The figure shows three views and two pictorial views of one solid part (mm, origin at its lowest corner). Answer the questions. A direction names the side the tool comes from. Coordinates: 2 decimals unless noted, no trailing zeros. Loops run counter-clockwise (first coordinate to the right, second up) from the corner with the lowest first, then second, coordinate; pieces in that order, holes last. Notation, with made-up numbers: M -20.75,65.5 L 6.25,65.5 A28 cw 6.25,89.5 Z; hole C -4,6.25 d9. An arc over 180 degrees is marked long. Return JSON: item names as keys, results as strings. Group by question number.
1. The mould has two halves that part along X. Classify the marked faces 1, 2 and 3: pulls with the +X half, pulls with the -X half, needs draft (parallel to the pull), parting line crosses it, or undercut.
2. Which of the six approach directions +Z, -Z, +X, -X, +Y, -Y give full straight-line access (tool end or side, diameter ignored) to the marked faces 4, 5, 6, 7 and 8?
3. Straight lines are drawn through the part: L1, parallel to X at y = 5.75, z = 1 (1 decimal); L2, parallel to Z at x = 3, y = 4.75; L3, parallel to Y at x = 9.75, z = 3. For each, find the intervals that lie inside material, in ascending order. Write a range as from..to.
4. Given P1, Ø1.6, axis at x = 1.5, z = 6, coming from the +Y side; P2, Ø4, axis at x = 14.5, z = 1, coming from the -Y side; P3, Ø3, axis at x = 6.5, y = 2.5, coming from the -Z side; P4, Ø5, axis at x = 21, z = 6.5, coming from the +Y side (1 decimal), each flat-ended and moving along its own axis, determine where each tip first touches the part or whether it passes through.
5. Section C-C (x = 8.25) is taken. Write down the section's boundary in (y, z), then the cut area to 3 significant figures.
6. Section B-B (z = 7) is taken. Write down the section's boundary in (x, y) (1 decimal).
7. Section D-D (y = 1.75) is taken. Write down the section's boundary in (x, z) (1 decimal), then the cut area to 3 significant figures.
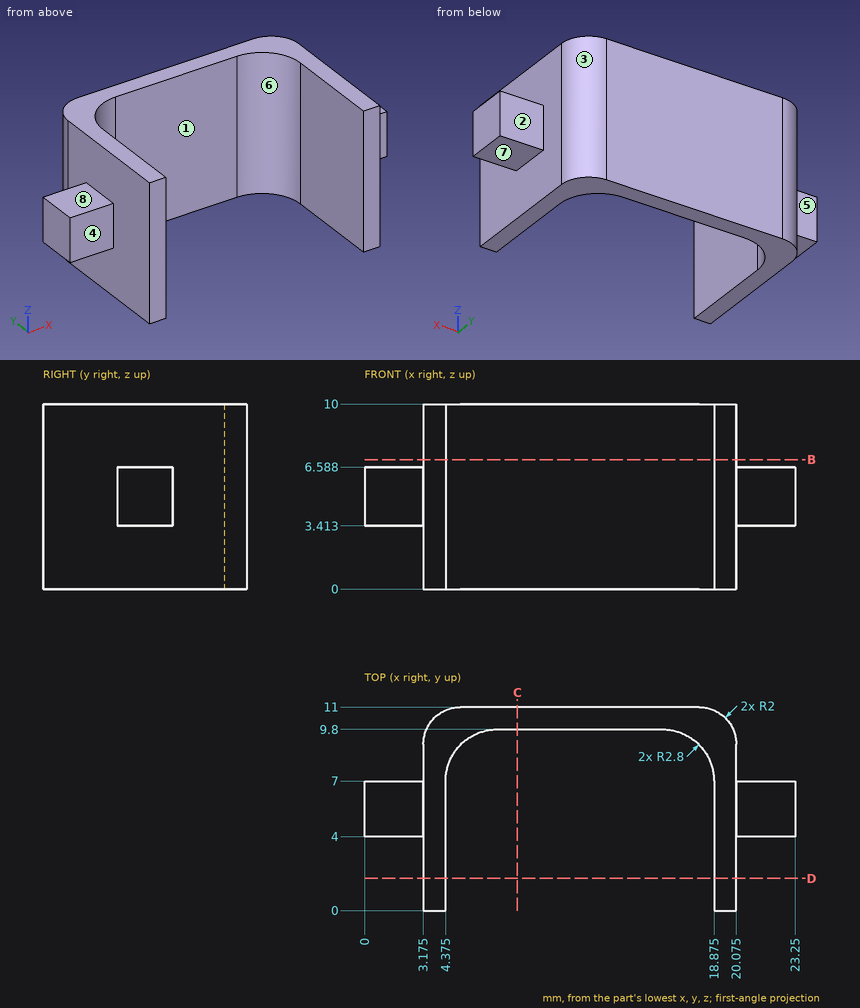
Worked out:
{
 "1": {"face 1": "undercut", "face 2": "needs draft", "face 3": "pulls with the +X half"},
 "2": {"face 4": "+Z, -Z, -X, -Y", "face 5": "+Z, -Z, -X, +Y", "face 6": "+Z, -Z, -Y", "face 7": "-Z, +X, +Y, -Y", "face 8": "+Z, -X, +Y, -Y"},
 "3": {"L1": "3.2..4.4, 18.9..20.1", "L2": "3.41..6.59", "L3": "9.8..11"},
 "4": {"P1": "y = 7", "P2": "y = 9.77", "P3": "through", "P4": "y = 11"},
 "5": {"outline": "M 9.8,0 L 11,0 L 11,10 L 9.8,10 Z", "area": "12.0 mm^2"},
 "6": {"outline": "M 3.2,0 L 4.4,0 L 4.4,7 A2.8 cw 7.2,9.8 L 16.1,9.8 A2.8 cw 18.9,7 L 18.9,0 L 20.1,0 L 20.1,9 A2 ccw 18.1,11 L 5.2,11 A2 ccw 3.2,9 Z"},
 "7": {"outline": "M 3.2,0 L 4.4,0 L 4.4,10 L 3.2,10 Z; M 18.9,0 L 20.1,0 L 20.1,10 L 18.9,10 Z", "area": "24.0 mm^2"}
}
